```python
from build123d import *

# Parameters (mm, degrees)
SKETCH_1_R          = 3
EXTRUDE_1_DEPTH     = 15
SKETCH_2_R          = 5
CUT_EXTRUDE_1_DEPTH = 6
SKETCH_3_R          = 5
CUT_EXTRUDE_2_DEPTH = 3
SKETCH_4_R          = 2.5
CUT_EXTRUDE_3_DEPTH = 10


with BuildPart() as part:
    # 草图1 → 凸台-拉伸1 (new body)
    with BuildSketch(Plane.XY):
        with BuildLine():
            Line((0, 0), (30, 0))
            Line((30, 0), (30, -20))
            Line((30, -20), (0, -20))
            Line((0, -20), (-20.06938155, -14.664278475))
            ThreePointArc((-20.06938155, -14.664278475), (-27.106051537, -2.220832162), (-14.512363219, 4.543271266))
            Line((-14.512363219, 4.543271266), (0, 0))
        make_face()
        with Locations((7.5, -10)):
            Circle(SKETCH_1_R, mode=Mode.SUBTRACT)
        with Locations((22.5, -10)):
            Circle(SKETCH_1_R, mode=Mode.SUBTRACT)
    extrude(amount=EXTRUDE_1_DEPTH)

    # 草图2 → 切除-拉伸1 (cut)
    with BuildSketch(Plane.XY.offset(15)):
        with Locations((7.5, -10)):
            Circle(SKETCH_2_R)
        with Locations((22.5, -10)):
            Circle(SKETCH_2_R)
    extrude(amount=-CUT_EXTRUDE_1_DEPTH, mode=Mode.SUBTRACT)

    # 草图3 → 切除-拉伸2 (cut)
    with BuildSketch(Plane(origin=(0, 0, 0), x_dir=(-1, 0, 0), z_dir=(0, 0, -1))):
        with Locations((17.5, -5)):
            Circle(SKETCH_3_R)
    extrude(amount=-CUT_EXTRUDE_2_DEPTH, mode=Mode.SUBTRACT)

    # 草图4 → 切除-拉伸3 (cut)
    with BuildSketch(Plane(origin=(0, 0, 3), x_dir=(-1, 0, 0), z_dir=(0, 0, -1))):
        with Locations((17.5, -5)):
            Circle(SKETCH_4_R)
    extrude(amount=-CUT_EXTRUDE_3_DEPTH, mode=Mode.SUBTRACT)


solid = part.part
```
Here's how the part is built. I have some questions about the finished solid (model axes, mm). A direction names the side the tool comes from. Coordinates: 2 decimals unless noted, no trailing zeros. Order: outer loops, then holes, each group sorted by start corner. A loop starts at its lowest first (then second) coordinate and runs counter-clockwise, first axis right, second up.
1) I need wall thicknesses on line 1 (Y direction, x = 22.5, z = 13.05); line 2 (X direction, y = -12.5, z = 4.5); line 3 (Y direction, x = 7.5, z = 5.5). Which ranges of each line are inside material? Lowest first, please.
2) Will these pins go through, and if not, where does the flat tip stop? pin 1 (1 mm diameter, centred on y = -9.5, z = 6, fed in from -X); pin 2 (4 mm diameter, centred on x = -16.5, z = 10, fed in from +Y); pin 3 (9 mm diameter, centred on x = -17.5, y = -5, fed in from -Z); pin 4 (6 mm diameter, centred on x = 22, z = 11, fed in from +Y).
3) We'd pull the mould along Y, two halves only. Please class faces 1 (the face through (2, -7, 0)), 2 (the face through (-9.89, -17.37, 7.4)), 3 (the face through (17.505, -9.78, 12.042)): +Y half, -Y half, draft (parallel to the pull), parting line (faces both ways), or undercut.
4) Which directions (+Z, -Z, +X, -X, +Y, -Y) give clear straight access to the entire face, cutting with the end or side of a thin tool? Please do faces 4 (the face through (12.27, -8.5, 12.04)), 5 (the face through (15, 0, 7)), 6 (the face through (-13.5, -8, 1.5)).
5) Imagine slicing it at B-B on x = 7.5. List the corners of the cut face in (y, z) for me.
6) Imagine slicing it at A-A on z = 1.25. List the corners of the cut face in (x, y) for me, and give its area (3 significant figures).
7) Imagine slicing it at D-D on y = -3.25. List the corners of the cut face in (x, z) for me, and give its area (3 significant figures).
8) Imagine slicing it at C-C on x = -17.5. List the corners of the cut face in (y, z) for me, and give its area (3 significant figures).
Response values:
1. line 1: y = -20 to -15, -5 to 0
1. line 2: x = -24.11 to 5.84, 9.16 to 20.84, 24.16 to 30
1. line 3: y = -20 to -13, -7 to 0
2. pin 1: stops at x = -26.67
2. pin 2: stops at y = 5
2. pin 3: stops at z = 3
2. pin 4: stops at y = 0
3. face 1: draft
3. face 2: -Y half
3. face 3: undercut
4. face 4: +Z
4. face 5: +Z, -Z, +X, +Y
4. face 6: -Z
5. outline: (-20, 0) - (-13, 0) - (-13, 9) - (-15, 9) - (-15, 15) - (-20, 15) - close; (-7, 0) - (0, 0) - (0, 15) - (-5, 15) - (-5, 9) - (-7, 9) - close
6. outline: (-20.07, -14.66) - (0, -20) - (30, -20) - (30, 0) - (0, 0) - (-14.51, 4.54) arc R10 ccw (long way) to start; hole circle Ø10 at (-17.5, -5); hole circle Ø6 at (7.5, -10); hole circle Ø6 at (22.5, -10)
6. area: 979 mm2
7. outline: (-27.35, 0) - (-22.18, 0) - (-22.18, 3) - (-19.29, 3) - (-19.29, 13) - (-15.71, 13) - (-15.71, 3) - (-12.82, 3) - (-12.82, 0) - (30, 0) - (30, 15) - (-27.35, 15) - close
7. area: 796 mm2
8. outline: (-15.35, 0) - (-10, 0) - (-10, 3) - (-7.5, 3) - (-7.5, 13) - (-2.5, 13) - (-2.5, 3) - (0, 3) - (0, 0) - (5, 0) - (5, 15) - (-15.35, 15) - close
8. area: 225 mm2
